Drawing for the job (mm, zero at the part's lowest x, y, z). A direction names the side the tool comes from. Coordinates: 2 decimals unless noted, no trailing zeros. Write each loop counter-clockwise with the first axis right and the second up, starting at its lowest first coordinate (ties: lowest second). Pieces come first, ordered by that corner, then holes. Notation, with made-up numbers: M -25,-30 L 24,-30 A16 ccw 24,-22 Z; hole C 72.5,-4.75 d1. An arc over 180 degrees is marked long. Put each result on its own line as item: value. Start each with the question number.
Q1. Which spindle directions (+Z, -Z, +X, -X, +Y, -Y) get a long thin tool onto all of the face, cutting with end or side? Do the marked faces 4 and 5. Say none if no direction does.
Q2. Drop flat-ended pins along their axis: pin 1 (5.5 mm diameter, centred on x = 34.14, z = 60.34, fed in from -Y); pin 2 (1 mm diameter, centred on y = 2.5, z = 43.5, fed in from -X); pin 3 (8 mm diameter, centred on y = 19.5, z = 34.5, fed in from -X); pin 4 (5 mm diameter, centred on x = 9, y = 7.5, fed in from -Z) (1 decimal). Give the stop position or say it passes through.
Q3. Pull direction Z, two halves, no side cores. Call the marked faces 1, 2 and 3: pulls with the +Z half, pulls with the -Z half, needs draft (parallel to the pull), parting line crosses it, or undercut.
Q4. Drill centre lines: line 1 along Z through (x, y) = (55, 3.5) (1 decimal); line 2 along X through (y, z) = (12, 46.5) (1 decimal); line 3 along X through (y, z) = (1.5, 40). Where is each one in solid material? Low to high.
Q5. Cut at B-B (y = 2.5). Give the number of separate pieces and of enclosed holes in the cut face, then the cut area to 3 significant figures.
Q6. Cut at D-D (x = 6). Write the cut outline in (y, z) (1 decimal), then the cut area to 3 significant figures.
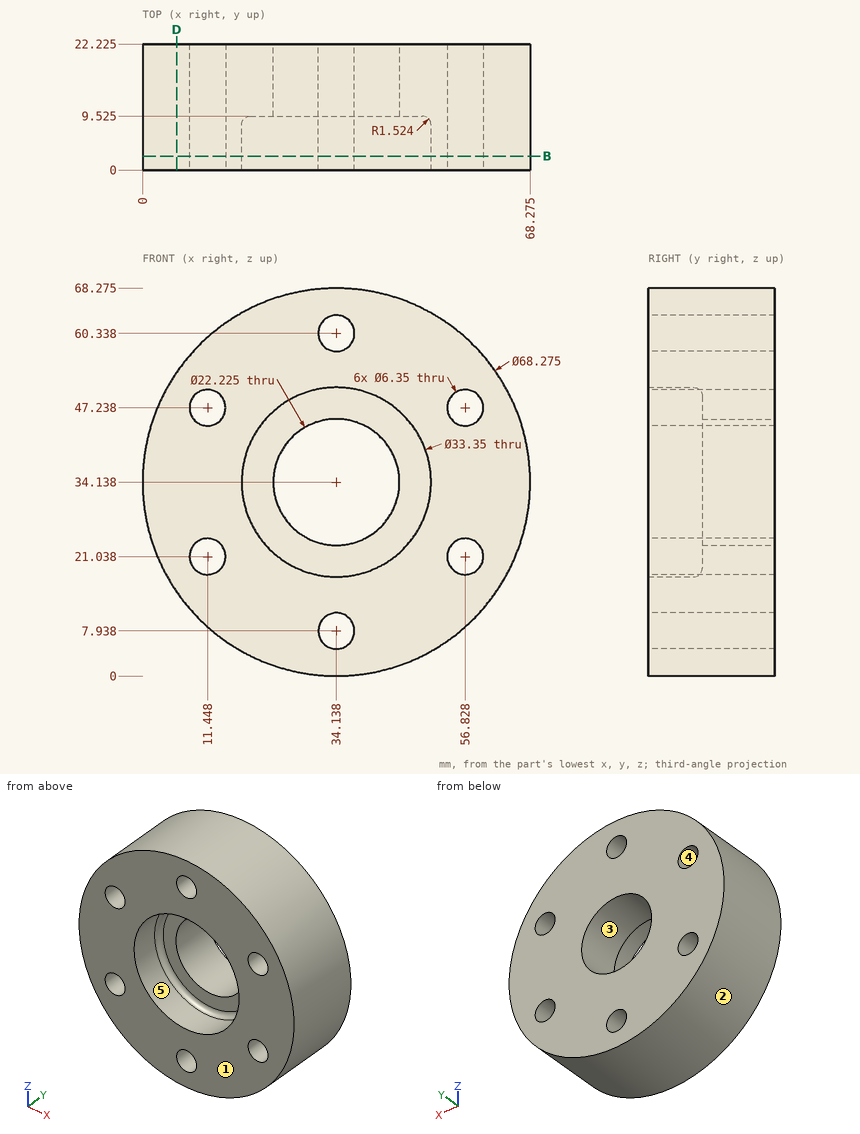
Computed values:
1. face 4: +Y, -Y
1. face 5: -Y
2. pin 1: through
2. pin 2: x = 1.17
2. pin 3: x = 0
2. pin 4: z = 8.6
3. face 1: needs draft
3. face 2: parting line crosses it
3. face 3: undercut
4. line 1: 7.1 to 18.4, 23.6 to 44.6, 49.8 to 61.2
4. line 2: 2.3 to 8.4, 14.5 to 53.7, 59.9 to 66
4. line 3: 0.51 to 18.53, 49.75 to 67.77
5. separate pieces: 1
5. enclosed holes: 7
5. area: 2,600 mm2
6. outline: M 0,14.8 L 22.2,14.8 L 22.2,53.5 L 0,53.5 Z
6. area: 859 mm2
